from build123d import *

# Parameters (mm, degrees)
CROQUIS3_W            = 2.449489742
CROQUIS3_H            = 1
CORTAR_EXTRUIR1_DEPTH = 5
CROQUIS4_R            = 1.5
CORTAR_EXTRUIR2_DEPTH = 2
CROQUIS6_R            = 2.6
CORTAR_EXTRUIR3_DEPTH = 0.7
CORTAR_EXTRUIR4_DEPTH = 0.5


with BuildPart() as part:
    # Croquis1 → Revolución1 (revolve)
    with BuildSketch(Plane.XY, mode=Mode.PRIVATE) as revoluci_n1_sk:
        with BuildLine():
            Line((0, 0), (0, 1.75))
            Line((0, 1.75), (-1, 1.75))
            Line((-1, 1.75), (-1, 12.2))
            Line((-1, 12.2), (-29.3, 12.2))
            ThreePointArc((-29.3, 12.2), (-30.360660172, 11.760660172), (-30.8, 10.7))
            Line((-30.8, 10.7), (-30.8, 0))
            Line((-30.8, 0), (0, 0))
        make_face()
    revolve(revoluci_n1_sk.sketch.rotate(Axis((-226.683028939, 0, 0), (1, 0, 0)), 90), axis=Axis((-226.683028939, 0, 0), (1, 0, 0)))

    # Croquis2 → Revolución2 (revolve)
    with BuildSketch(Plane.XY, mode=Mode.PRIVATE) as revoluci_n2_sk:
        with BuildLine():
            Line((-57, 12.5), (-31.6, 12.5))
            ThreePointArc((-31.6, 12.5), (-31.034314575, 12.265685425), (-30.8, 11.7))
            Line((-30.8, 11.7), (-30.8, 0))
            Line((-30.8, 0), (-69.3, 0))
            Line((-69.3, 0), (-69.3, 1.75))
            Line((-69.3, 1.75), (-60.3, 1.75))
            Line((-60.3, 1.75), (-60.3, 3.5))
            Line((-60.3, 3.5), (-57.8, 3.5))
            Line((-57.8, 3.5), (-57.8, 11.7))
            ThreePointArc((-57.8, 11.7), (-57.565685425, 12.265685425), (-57, 12.5))
        make_face()
    revolve(revoluci_n2_sk.sketch.rotate(Axis((-1000, 0, 0), (1, 0, 0)), 90), axis=Axis((-1000, 0, 0), (1, 0, 0)))

    # Croquis3 → Cortar-Extruir1 (cut)
    with BuildSketch(Plane.ZY.offset(69.3)):
        with Locations((0, 1.75)):
            Rectangle(CROQUIS3_W, CROQUIS3_H)
    extrude(amount=-CORTAR_EXTRUIR1_DEPTH, mode=Mode.SUBTRACT)

    # Croquis4 → Cortar-Extruir2 (cut)
    with BuildSketch(Plane.ZY.offset(57.8)):
        with Locations((-8.5, 0)):
            Circle(CROQUIS4_R)
        with Locations((8.5, 0)):
            Circle(CROQUIS4_R)
    extrude(amount=-CORTAR_EXTRUIR2_DEPTH, mode=Mode.SUBTRACT)

    # Croquis6 → Cortar-Extruir3 (cut)
    with BuildSketch(Plane.ZY.offset(57.8)):
        with Locations((0, 8)):
            Circle(CROQUIS6_R)
        with Locations(Location((0, -8, 0), (0, 0, 180))):
            Circle(CROQUIS6_R)
    extrude(amount=-CORTAR_EXTRUIR3_DEPTH, mode=Mode.SUBTRACT)

    # Croquis7 → Cortar-Extruir4 (cut)
    with BuildSketch(Plane.ZY.offset(57.1)):
        Polygon((0.2, 9.9), (-0.2, 9.9), (-0.2, 8.2), (-1.9, 8.2), (-1.9, 7.8), (-0.2, 7.8), (-0.2, 6.1), (0.2, 6.1), (0.2, 7.8), (1.9, 7.8), (1.9, 8.2), (0.2, 8.2), align=None)
        Polygon((-0.2, -7.8), (-1.9, -7.8), (-1.9, -8.2), (-0.2, -8.2), (-0.2, -9.9), (0.2, -9.9), (0.2, -8.2), (1.9, -8.2), (1.9, -7.8), (0.2, -7.8), (0.2, -6.1), (-0.2, -6.1), align=None)
    extrude(amount=-CORTAR_EXTRUIR4_DEPTH, mode=Mode.SUBTRACT)


solid = part.part
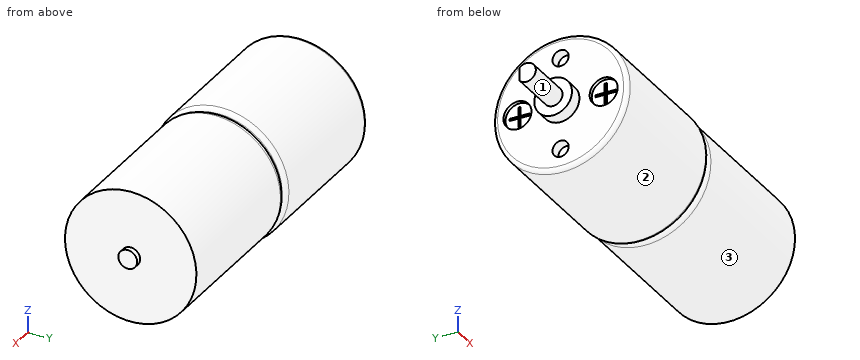
Design review of the part built by this model. Coordinates are the model's own, in mm. Face numbers are marked on the shaded views. A direction names the side the tool comes from. Coordinates: 2 decimals unless noted, no trailing zeros. Loops run counter-clockwise (first coordinate to the right, second up) from the corner with the lowest first, then second, coordinate; pieces in that order, holes last. Notation, with made-up numbers: (10.5, 39.5) -> (49.5, 39.5) arc R14 cw to (49.5, 63.5) -> close; hole circle Ø1 at (74.25, 62.5). An arc over 180 degrees is marked (long way). Use a Markdown table: item, result. Add a question column.
Item 1: We need section C-C, the plane x = -42.5. Write out the cut boundary in (y, z), and give its area (3 significant figures).
Item 2: Wall thickness on L1, parallel to X at y = -8, z = -3.5; L2, parallel to Y at x = -57.35, z = 0; L3, parallel to Y at x = -56.95, z = 8.5: over which ranges is each line inside the solid? List them lowest first. Write a range as from..to.
Item 3: Machinability: for the marked faces 1, 2 and 3, which of the approach directions +Z, -Z, +X, -X, +Y, -Y give a long, thin tool a straight path to every point of the face, cutting with its end or side? Answer none if there is none.
Item 4: Clearance check with flat-ended pins moving along their axes: P1, Ø8, axis at y = 2, z = 9, coming from the +X side; P2, Ø10, axis at x = -11.5, y = -9.5, coming from the +Z side; P3, Ø10, axis at y = -8.5, z = 4.5, coming from the -X side; P4, Ø12, axis at x = -48.5, z = -3, coming from the -Y side. State where each tip first meets the part, or that it passes through.
Item 5: We need section B-B, the plane x = -6. Write out the cut boundary in (y, z).
Numbers:
| question | item | result |
|---|---|---|
| 1 | outline | circle Ø25 at (0, 0) |
| 1 | area | 491 mm^2 |
| 2 | L1 | x = -57.8..-1 |
| 2 | L2 | y = -12.42..-10.6, -5.4..5.4, 10.6..12.42 |
| 2 | L3 | y = -9.17..-1.5, 1.5..9.17 |
| 3 | face 1 | -X |
| 3 | face 2 | +X, -X |
| 3 | face 3 | +X |
| 4 | P1 | stops at x = -1 |
| 4 | P2 | stops at z = 11.34 |
| 4 | P3 | stops at x = -57.8 |
| 4 | P4 | stops at y = -12.5 |
| 5 | outline | circle Ø24.4 at (0, 0) |
